from build123d import *

# Parameters (mm, degrees)
SKETCH1_W           = 211.1375
SKETCH1_H           = 33.3375
BOSS_EXTRUDE1_DEPTH = 3.175
BOSS_EXTRUDE2_DEPTH = 15.875
CUT_EXTRUDE1_REACH  = 216.6
FILLET1_R           = 1.27


with BuildPart() as part:
    # Sketch1 → Boss-Extrude1 (new body)
    with BuildSketch(Plane.XY):
        with Locations((105.56875, 16.66875)):
            Rectangle(SKETCH1_W, SKETCH1_H)
    extrude(amount=BOSS_EXTRUDE1_DEPTH)

    # Sketch2 → Boss-Extrude2 (add)
    with BuildSketch(Plane.XY.offset(3.175)):
        Polygon((5.08, 0), (5.08, 3.175), (3.175, 3.175), (3.175, 30.1625), (207.9625, 30.1625), (207.9625, 3.175), (206.0575, 3.175), (206.0575, 0), (211.1375, 0), (211.1375, 33.3375), (0, 33.3375), (0, 0), align=None)
    extrude(amount=BOSS_EXTRUDE2_DEPTH)

    # Sketch3 → Cut-Extrude1 (cut, up to next)
    with BuildSketch(Plane.XZ, mode=Mode.PRIVATE) as cut_extrude1_sk1:
        Polygon((207.9625, 3.175), (206.0575, 3.175), (206.0575, 9.525), (207.9625, 7.62), align=None)
    cut_extrude1_tool1 = extrude(cut_extrude1_sk1.sketch, amount=-CUT_EXTRUDE1_REACH, mode=Mode.PRIVATE) & part.part
    # Sketch3 → Cut-Extrude1 (cut, up to next)
    with BuildSketch(Plane.XZ, mode=Mode.PRIVATE) as cut_extrude1_sk2:
        Polygon((5.08, 9.525), (3.175, 7.62), (3.175, 3.175), (5.08, 3.175), align=None)
    cut_extrude1_tool2 = extrude(cut_extrude1_sk2.sketch, amount=-CUT_EXTRUDE1_REACH, mode=Mode.PRIVATE) & part.part
    add(cut_extrude1_tool1.solids().sort_by_distance((206.953971, 0, 5.901765))[0], mode=Mode.SUBTRACT)
    add(cut_extrude1_tool2.solids().sort_by_distance((4.183529, 0, 5.901765))[0], mode=Mode.SUBTRACT)

    # Fillet1
    fillet1_edges = [part.edges().sort_by_distance(p)[0] for p in [
        (105.56875, 0, 0),
        (211.1375, 16.66875, 0),
        (105.56875, 33.3375, 0),
        (0, 16.66875, 0),
        (0, 0, 9.525),
        (211.1375, 0, 9.525),
        (211.1375, 33.3375, 9.525),
        (0, 33.3375, 9.525),
    ]]
    fillet(fillet1_edges, radius=FILLET1_R)


solid = part.part
Design review of the part built by this model. Coordinates are the model's own, in mm. Coordinates: 2 decimals unless noted, no trailing zeros. Loops run counter-clockwise (first coordinate to the right, second up) from the corner with the lowest first, then second, coordinate; pieces in that order, holes last.
Item 1: Wall thickness on L1, parallel to X at y = 12.5, z = 10 (1 decimal); L2, parallel to Z at x = 113, y = 4 (3 decimals); L3, parallel to Y at x = 29.5, z = 4.25: over which ranges is each line inside the solid? List them lowest first.
Completed:
L1: x = 0 to 3.2, 208 to 211.1
L2: z = 0 to 3.175
L3: y = 30.16 to 33.34
Item 2: Clearance check with flat-ended pins moving along their axes: pin 1 (1.6 mm diameter, centred on y = 1, z = 14, fed in from +X); pin 2 (3 mm diameter, centred on x = 99, y = 22, fed in from +Z) (3 decimals); pin 3 (8 mm diameter, centred on x = 95.5, z = 11, fed in from -Y). State where each tip first meets the part, or that it passes through.
Completed:
pin 1: stops at x = 211.14
pin 2: stops at z = 3.175
pin 3: stops at y = 30.16
Item 3: Add section D-D (z = 5.5). Write out the cut boundary in (x, y) (1 decimal), and give its area (3 significant figures).
Completed:
outline: (0, 1.3) arc R1.3 ccw to (1.3, 0) - (3.2, 0) - (3.2, 30.2) - (208, 30.2) - (208, 0) - (209.9, 0) arc R1.3 ccw to (211.1, 1.3) - (211.1, 32.1) arc R1.3 ccw to (209.9, 33.3) - (1.3, 33.3) arc R1.3 ccw to (0, 32.1) - close
area: 861 mm2
Item 4: Add section A-A (z = 16). Write out the cut boundary in (x, y) (1 decimal), and give its area (3 significant figures).
Completed:
outline: (0, 1.3) arc R1.3 ccw to (1.3, 0) - (5.1, 0) - (5.1, 3.2) - (3.2, 3.2) - (3.2, 30.2) - (208, 30.2) - (208, 3.2) - (206.1, 3.2) - (206.1, 0) - (209.9, 0) arc R1.3 ccw to (211.1, 1.3) - (211.1, 32.1) arc R1.3 ccw to (209.9, 33.3) - (1.3, 33.3) arc R1.3 ccw to (0, 32.1) - close
area: 873 mm2
Item 5: Draft analysis for pull direction X (two halves, no side actions). For faces 1 (the flat face through (0, 17, 10)), 2 (the flat face through (3.175, 15, 11)), 3 (the flat face through (90, 0, 3)), 4 (the flat face through (211.138, 16, 10)), state which applies: pulls with the +X half, pulls with the -X half, needs draft (parallel to the pull), parting line crosses it, or undercut.
Completed:
face 1: pulls with the -X half
face 2: undercut
face 3: needs draft
face 4: pulls with the +X half
